Model file for the job. Use its own axes, mm. A direction names the side the tool comes from. Coordinates: 2 decimals unless noted, no trailing zeros. Write each loop counter-clockwise with the first axis right and the second up, starting at its lowest first coordinate (ties: lowest second). Pieces come first, ordered by that corner, then holes. Notation, with made-up numbers: M 86.25,58.25 L 111.25,58.25 A18 ccw 111.25,86.25 Z; hole C -25,20 d10. An arc over 180 degrees is marked long. One line per question, with ' | ' between items. Start each with the question number.
(1) Cut at A-A (z = 11.5). Write the cut outline in (x, y).
(2) Cut at D-D (x = 47.5). Write the cut outline in (y, z).
(3) Cut at B-B (x = 14). Write the cut outline in (y, z).
(4) Cut at C-C (y = -6.5). Write the cut outline in (x, z).
(5) Tool access for faces 1 (the face through (0, -5, 22.25)), 2 (the face through (22.25, -5, 9)), 3 (the face through (-20.75, -5, 0)): list every direction of +Z, -Z, +X, -X, +Y, -Y with a clear straight run to the whole face (end or side of a thin tool).
(6) Two-plate mould, pull along X, no slides. Class faces 4 (the face through (60, -5, -23)), 5 (the face through (0, -5, 20.75)), 6 (the face through (-4, -5, -22.25)): +X half, -X half, draft (parallel to the pull), parting line (faces both ways), or undercut.
(7) Wall check: probe 1 along X at (y, z) = (-5.5, 2.5). Give the ranges that are in metal, low to high.
(8) Flat gauge pin, fed straight in: pin 1 Ø1 at (x, y) = (1.5, -6.5) entering from -Z. Where does the tip first touch, or does it go through?
from build123d import *

# Parameters (mm, degrees)
F0_W        = 44.5
F0_H        = 44.5
F1_DEPTH    = 10
F2_W        = 41.5
F2_H        = 41.5
F3_DEPTH    = 10
F5_START    = 20
F4_W        = 10
F4_H        = 6
F5_DEPTH    = 40
F6_W        = 18.9917886164
F6_H        = 12.0773017406
F7_DEPTH    = 25
F8_R        = 15
F9_T1_DEPTH = 10


# Not quite as in the source:
# - a fillet or chamfer that OpenCascade refuses, or shapes differently, is made with other operations: its cross-section is extruded or revolved along the edge and cut away or added


with BuildPart() as f1:
    # F0 (on Front) → F1 (new body)
    with BuildSketch(Plane.XZ):
        Rectangle(F0_W, F0_H)
    extrude(amount=F1_DEPTH)

    # F2 (on Front) → F3 (cut)
    with BuildSketch(Plane.XZ):
        Rectangle(F2_W, F2_H)
    extrude(amount=F3_DEPTH, mode=Mode.SUBTRACT)

    # F4 (on Right) → F5 (join)
    with BuildSketch(Plane.YZ.offset(F5_START)):
        with Locations((-5, -22.75)):
            Rectangle(F4_W, F4_H)
    extrude(amount=F5_DEPTH)

    # F6 (on Front) → F7 (cut)
    with BuildSketch(Plane.XZ):
        with Locations((11.2541056918, -14.7113491297)):
            Rectangle(F6_W, F6_H)
    extrude(amount=F7_DEPTH, mode=Mode.SUBTRACT)

    # F8
    f8_edges = [f1.edges().sort_by_distance(p)[0] for p in [
        (22.25, -5, -19.75),
    ]]
    fillet(f8_edges, radius=F8_R)

    # F9: fillet of radius 5 on 1 edges, made by hand

    # F9_s2 → F9_t1 (join)
    with BuildSketch(Plane.XZ):
        with BuildLine():
            ThreePointArc((20, -25.75), (18.1883438845, -23.2188711259), (15.2303039929, -22.25))
            Line((15.2303039929, -22.25), (20, -22.25))
            Line((20, -22.25), (20, -25.75))
        make_face()
    extrude(amount=F9_T1_DEPTH)


solid = f1.part
Filled in:
1) outline: M -22.25,-10 L -20.75,-10 L -20.75,0 L -22.25,0 Z; M 20.75,-10 L 22.25,-10 L 22.25,0 L 20.75,0 Z
2) outline: M -10,-25.75 L 0,-25.75 L 0,-19.75 L -10,-19.75 Z
3) outline: M -10,-22.25 L 0,-22.25 L 0,-20.75 L -10,-20.75 Z; M -10,20.75 L 0,20.75 L 0,22.25 L -10,22.25 Z
4) outline: M -22.25,-22.25 L 15.23,-22.25 A5 cw 20,-25.75 L 60,-25.75 L 60,-19.75 L 37.25,-19.75 A15 cw 22.25,-4.75 L 22.25,22.25 L -22.25,22.25 Z; hole M -20.75,-20.75 L 20.75,-20.75 L 20.75,20.75 L -20.75,20.75 Z
5) face 1: +Z, +X, -X, +Y, -Y | face 2: +Z, +X, +Y, -Y | face 3: +Y, -Y
6) face 4: +X half | face 5: undercut | face 6: draft
7) probe 1: -22.25 to -20.75, 20.75 to 22.25
8) pin 1: z = -22.25
